Part model, mm, in its own coordinate system. A direction names the side the tool comes from. Give positions to 0.01 mm unless a question says otherwise; leave off trailing zeros. Order: outer loops, then holes, each group sorted by start corner. A loop starts at its lowest first (then second) coordinate and runs counter-clockwise, first axis right, second up. Notation, with made-up numbers: M 57.5,-1 L 71.5,-1 A26 ccw 71.5,32 Z; hole C -27.75,34.25 d5. An arc over 180 degrees is marked long. Answer as a JSON object with one key per item and string values.
from build123d import *

# Parameters (mm, degrees)
F1_R          = 10
F1_R_2        = 2.125
F2_DEPTH      = 70
F3_W          = 130.2564469211
F3_H          = 20
F3_W_2        = 25.4596173763
F3_W_3        = 28.8759171963
F4_DEPTH      = 100
F4_DEPTH_BACK = 100
F5_R          = 2.125
F6_DEPTH      = 70
F9_DEPTH      = 4


with BuildPart() as f2:
    # F1 (on Front) → F2 (new body)
    with BuildSketch(Plane.XZ):
        with BuildLine():
            Line((333.3, 0), (0, 0))
            Line((0, 0), (-40.7109649446, -7.1784415304))
            ThreePointArc((-40.7109649446, -7.1784415304), (-54.7650426184, -14.7715124925), (-61.4796391993, -29.2658568603))
            ThreePointArc((-61.4796391993, -29.2658568603), (-54.9671092091, -49.2553101365), (-35.6024128261, -57.4406521057))
            Line((-35.6024128261, -57.4406521057), (-25.606345873, -57.1602141095))
            ThreePointArc((-25.606345873, -57.1602141095), (-12.1544941746, -60.6052272274), (-2.5623294895, -70.6456856906))
            Line((-2.5623294895, -70.6456856906), (278.9276717153, -56.0849576382))
            Line((278.9276717153, -56.0849576382), (333.3, -35.7395332009))
            ThreePointArc((333.3, -35.7395332009), (351.1697666005, -17.8697666005), (333.3, 0))
        make_face()
        with Locations((-36.3127197699, -32.1221294279)):
            Circle(F1_R, mode=Mode.SUBTRACT)
        with Locations((333.3, -17.8697666005)):
            Circle(F1_R, mode=Mode.SUBTRACT)
        with BuildLine():
            Line((-40.7109649446, -7.1784415304), (0, 0))
            Line((0, 0), (-51.8790856004, 3.4624293912))
            Line((-51.8790856004, 3.4624293912), (-93.7052443624, -3.4624293912))
            Line((-93.7052443624, -3.4624293912), (-61.4796391993, -29.2658568603))
            ThreePointArc((-61.4796391993, -29.2658568603), (-54.7650426184, -14.7715124925), (-40.7109649446, -7.1784415304))
        make_face()
        with Locations((-68.2217553258, -8.4483278915)):
            Circle(F1_R_2, mode=Mode.SUBTRACT)
    extrude(amount=F2_DEPTH)

    # F3 (on Top) → F4 (cut, two sides)
    with BuildSketch(Plane.XY) as f4_sk:
        with Locations((-76.2078319233, -35)):
            Rectangle(F3_W, F3_H)
        with Locations((346.1741060019, -35)):
            Rectangle(F3_W_2, F3_H)
        with Locations((319.0063387156, -35)):
            Rectangle(F3_W_3, F3_H)
    extrude(amount=F4_DEPTH, mode=Mode.SUBTRACT)
    extrude(f4_sk.sketch, amount=-F4_DEPTH_BACK, mode=Mode.SUBTRACT)

    # F5 (on Front) → F6 (join)
    with BuildSketch(Plane.XZ):
        with BuildLine():
            Line((213.3, 0), (233.3, 0))
            ThreePointArc((233.3, 0), (213.3, 20), (193.3, 0))
            Line((193.3, 0), (213.3, 0))
        make_face()
        with Locations((213.3, 10)):
            Circle(F5_R, mode=Mode.SUBTRACT)
    extrude(amount=F6_DEPTH)

    # F8 (on offset) → F9 (cut, symmetric)
    with BuildSketch(Plane.XZ.offset(35)):
        with BuildLine():
            Line((193.3, 0), (233.3, 0))
            ThreePointArc((233.3, 0), (213.3, 20), (193.3, 0))
        make_face()
    extrude(amount=F9_DEPTH, both=True, mode=Mode.SUBTRACT)


solid = f2.part
1. Cut at B-B on z = -51. Give the cut face in (x, y), plus the area to 3 significant figures.
Worked answers:
{"outline": "M -53.2,-70 L 292.52,-70 L 292.52,0 L -53.2,0 L -53.2,-25 L -11.08,-25 L -11.08,-45 L -53.2,-45 Z", "area": "23,400 mm^2"}
2. Cut at A-A on x = 203.5. Give the cut face in (y, z), plus the area to 3 significant figures.
Worked answers:
{"outline": "M -70,-59.99 L 0,-59.99 L 0,17.43 L -31,17.43 L -31,0 L -39,0 L -39,17.43 L -70,17.43 Z", "area": "5,280 mm^2"}
3. Pin check, flat tips, straight feed: P1, Ø22, axis at x = 208.5, z = 13, coming from the +Y side; P2, Ø6, axis at y = -37, z = -21.5, coming from the +X side; P3, Ø5, axis at x = 214, y = -28, coming from the -Z side; P4, Ø10, axis at y = -38.5, z = -23.5, coming from the -X side. Stop position of each tip, or through.
Worked answers:
{"P1": "stops at y = 0", "P2": "stops at x = 304.57", "P3": "stops at z = -59.57", "P4": "stops at x = -11.08"}
4. Cut at C-C on x = 113. Give the cut face in (y, z), plus the area to 3 significant figures.
Worked answers:
{"outline": "M -70,-64.67 L 0,-64.67 L 0,0 L -70,0 Z", "area": "4,530 mm^2"}
5. Which spindle directions (+Z, -Z, +X, -X, +Y, -Y) get a long thin tool onto all of the face, cutting with end or side? Do faces 4 (the cylindrical face through (342.84, -12.32, -14.87)), 5 (the flat face through (-11.08, -35, -31)). Say none if no direction does.
Worked answers:
{"face 4": "+Y, -Y", "face 5": "+Z, -Z, -X"}
6. Probe line 1 along Z through (x, y) = (333.3, -64.75); line 2 along X through (y, z) = (-38.5, -23); line 3 along X through (y, z) = (-22.5, -20.5). List the from-to ranges inside material, lowest first.
Worked answers:
{"line 1": "z = -35.74 to -27.87, -7.87 to 0", "line 2": "x = -11.08 to 304.57", "line 3": "x = -72.43 to 323.65, 342.95 to 350.98"}
7. Two-plate mould, pull along Y, no slides. Class faces 1 (the flat face through (299.692, -34.51, -48.315)), 2 (the flat face through (213, -31, 6)), 3 (the flat face through (126, -70, -25)): +Y half, -Y half, draft (parallel to the pull), parting line (faces both ways), or undercut.
Worked answers:
{"face 1": "draft", "face 2": "undercut", "face 3": "-Y half"}
